Print and shaded views of the part. All mm, measured from the part's lowest x, y and z. Round coordinates to 2 decimals unless told otherwise and drop trailing zeros. Loops run counter-clockwise (first coordinate to the right, second up) from the corner with the lowest first, then second, coordinate; pieces in that order, holes last. Notation, with made-up numbers: (40, 49.5) -> (44, 49.5) arc R20 cw to (44, 79.5) -> close; hole circle Ø8 at (-29.75, 0.25). An arc over 180 degrees is marked (long way). Use a Markdown table: item, result.
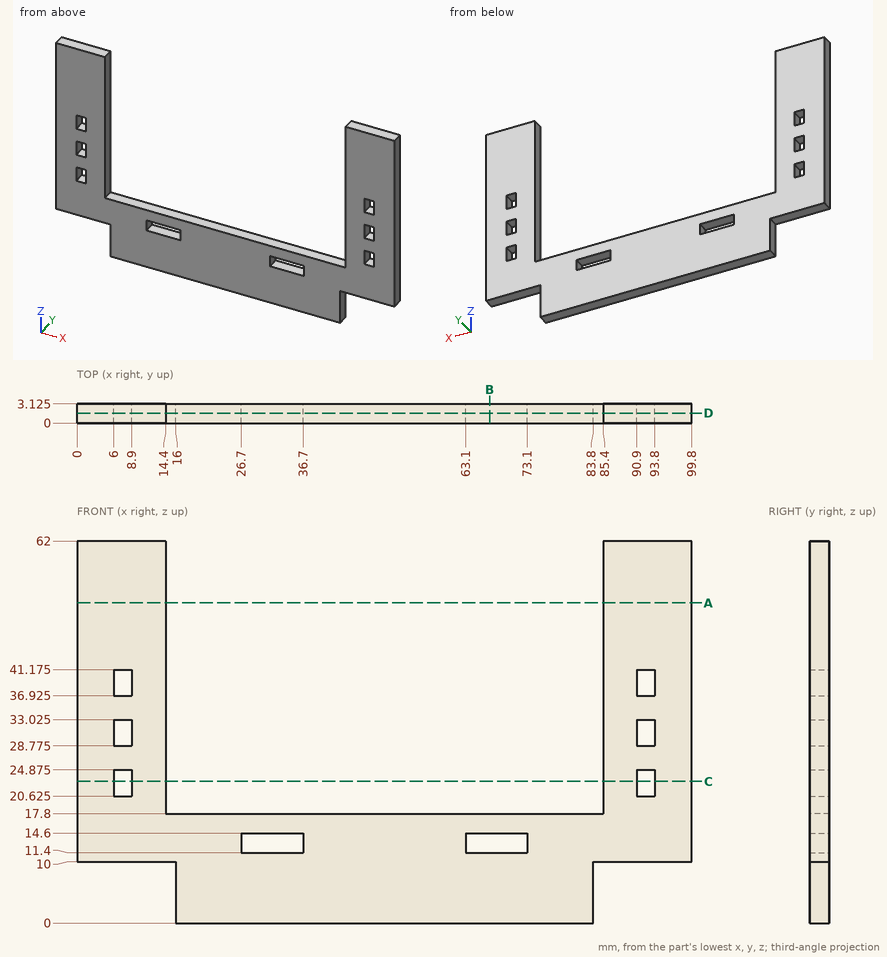
Q1. Drill centre lines: L1, parallel to X at y = 2, z = 30; L2, parallel to X at y = 2.2, z = 26.5; L3, parallel to Z at x = 66, y = 2.1. Where is each one in solid material? Low to high. Write a range as from..to.
Results list:
| item | result |
|---|---|
| L1 | x = 0..6, 8.9..14.4, 85.4..90.9, 93.8..99.8 |
| L2 | x = 0..14.4, 85.4..99.8 |
| L3 | z = 0..11.4, 14.6..17.8 |
Q2. Band-saw the part on A-A, the plane z = 52. Give the cut face in (x, y) (3 decimals).
Results list:
| item | result |
|---|---|
| outline | (0, 0) -> (14.4, 0) -> (14.4, 3.125) -> (0, 3.125) -> close; (85.4, 0) -> (99.8, 0) -> (99.8, 3.125) -> (85.4, 3.125) -> close |
Q3. Band-saw the part on B-B, the plane x = 67. Give the cut face in (y, z) (3 decimals).
Results list:
| item | result |
|---|---|
| outline | (0, 0) -> (3.125, 0) -> (3.125, 11.4) -> (0, 11.4) -> close; (0, 14.6) -> (3.125, 14.6) -> (3.125, 17.8) -> (0, 17.8) -> close |
Q4. Flat gauge pins, fed straight in: pin 1 (1.6 mm diameter, centred on x = 95.5, y = 1, fed in from -Z); pin 2 (4 mm diameter, centred on x = 77.5, z = 8.5, fed in from -Y); pin 3 (1 mm diameter, centred on x = 23, y = 2.5, fed in from +Z). Where does each tip first touch, or does it go through?
Results list:
| item | result |
|---|---|
| pin 1 | stops at z = 10 |
| pin 2 | stops at y = 0 |
| pin 3 | stops at z = 17.8 |
Q5. Band-saw the part on C-C, the plane z = 23. Give the cut face in (x, y) (3 decimals).
Results list:
| item | result |
|---|---|
| outline | (0, 0) -> (6, 0) -> (6, 3.125) -> (0, 3.125) -> close; (8.9, 0) -> (14.4, 0) -> (14.4, 3.125) -> (8.9, 3.125) -> close; (85.4, 0) -> (90.9, 0) -> (90.9, 3.125) -> (85.4, 3.125) -> close; (93.8, 0) -> (99.8, 0) -> (99.8, 3.125) -> (93.8, 3.125) -> close |
Q6. Band-saw the part on D-D, the plane y = 1.65. Give the number of separate pieces and of enclosed holes in the cut face, plus the area to 3 significant figures.
Results list:
| item | result |
|---|---|
| separate pieces | 1 |
| enclosed holes | 8 |
| area | 2,590 mm² |
